Read the model definition and answer for the solid it produces. Units are mm, in the model's axes. A direction names the side the tool comes from. Give positions to 0.01 mm unless a question says otherwise; leave off trailing zeros. Write each loop counter-clockwise with the first axis right and the second up, starting at its lowest first coordinate (ties: lowest second). Pieces come first, ordered by that corner, then holes. Notation, with made-up numbers: M 6,60.5 L 40,60.5 A31 ccw 40,87.5 Z; hole C 47.5,-39.75 d9. An arc over 180 degrees is marked long. Use a Markdown table: item, result. Add a question column.
Item 1: A cutting plane is placed at A-A on y = 0. Determine the outline of the cut face in (x, z).
Item 2: The mould has two halves that part along Y. Classify faces 1 (the flat face through (10, 1, 3)), 2 (the cylindrical face through (-0.867, -3.905, 9.479)): pulls with the +Y half, pulls with the -Y half, needs draft (parallel to the pull), parting line crosses it, or undercut.
Item 3: Consider probe 1 along Z at (x, y) = (-34.5, -7.5); probe 2 along X at (y, z) = (-21, 1.5); probe 3 along X at (y, z) = (-18.5, 2.25). Determine where each line is inside the solid, lowest interval first. Write a range as [from, to].
Item 4: For faces 3 (the cylindrical face through (5, 1.6, 5.5)), 4 (the flat face through (0, 0, 11)), determine the directions among +Z, -Z, +X, -X, +Y, -Y from which every point of the face is accessible in a straight line to the end or side of a thin tool.
Item 5: A cutting plane is placed at D-D on z = 4.75. Determine the outline of the cut face in (x, y), then the cut area to 3 significant figures.
Item 6: Given P1, Ø2, axis at x = -29, y = 28.5, coming from the +Z side; P2, Ø5, axis at x = -10, z = 1.5, coming from the +Y side; P3, Ø5, axis at x = -37.5, z = 3.5, coming from the -Y side, each flat-ended and moving along its own axis, determine where each tip first touches the part or whether it passes through.
Item 7: A cutting plane is placed at C-C on z = 9.75. Determine the outline of the cut face in (x, y), then the cut area to 3 significant figures.
from build123d import *

# Parameters (mm, degrees)
F0_R     = 50
F0_R_2   = 5.25
F1_DEPTH = 3
F0_R_3   = 4
F2_DEPTH = 8
F3_DEPTH = 11
F4_R     = 2


with BuildPart() as f1:
    # F0 (on Top) → F1 (new body)
    with BuildSketch(Plane.XY):
        Circle(F0_R)
        Circle(F0_R_2, mode=Mode.SUBTRACT)
    extrude(amount=F1_DEPTH)

    # F0 (on Top) → F2 (join)
    with BuildSketch(Plane.XY):
        Circle(F0_R_2)
        Circle(F0_R_3, mode=Mode.SUBTRACT)
    extrude(amount=F2_DEPTH)

    # F0 (on Top) → F3 (join)
    with BuildSketch(Plane.XY):
        Circle(F0_R_3)
    extrude(amount=F3_DEPTH)

    # F4
    f4_edges = [f1.edges().sort_by_distance(p)[0] for p in [
        (-50, 0, 3),
    ]]
    fillet(f4_edges, radius=F4_R)


solid = f1.part
Filled in:
| question | item | result |
|---|---|---|
| 1 | outline | M -50,0 L 50,0 L 50,1 A2 ccw 48,3 L 5.25,3 L 5.25,8 L 4,8 L 4,11 L -4,11 L -4,8 L -5.25,8 L -5.25,3 L -48,3 A2 ccw -50,1 Z |
| 2 | face 1 | needs draft |
| 2 | face 2 | parting line crosses it |
| 3 | probe 1 | [0, 3] |
| 3 | probe 2 | [-45.31, 45.31] |
| 3 | probe 3 | [-45.98, 45.98] |
| 4 | face 3 | +Z |
| 4 | face 4 | +Z, +X, -X, +Y, -Y |
| 5 | outline | C 0,0 d10.5 |
| 5 | area | 86.6 mm² |
| 6 | P1 | z = 3 |
| 6 | P2 | y = 49.43 |
| 6 | P3 | y = -34.83 |
| 7 | outline | C 0,0 d8 |
| 7 | area | 50.3 mm² |
